from build123d import *

# Parameters (mm, degrees)
F0_W      = 43.6
F0_H      = 122.8
F1_DEPTH  = 6.1
F2_T      = -2
F3_R      = 3.5
F3_R_2    = 1.3
F4_DEPTH  = 2.5
F5_DEPTH  = 2.001
F6_W      = 1.5
F6_H      = 108.8
F6_W_2    = 5
F7_DEPTH  = 2.5
F8_W      = 5
F8_H      = 10
F9_DEPTH  = 1.5
F10_W     = 3
F10_H     = 10
F11_DEPTH = 25
F11_TAPER = -10
F0_W_2    = 5.5
F12_DEPTH = 4
F14_DEPTH = 15
F16_W     = 10
F16_H     = 3.6
F17_DEPTH = 11


with BuildPart() as f1:
    # F0 (on Top) → F1 (new body)
    with BuildSketch(Plane.XY):
        with Locations((-27.3, 0)):
            Rectangle(F0_W, F0_H)
    extrude(amount=F1_DEPTH)

    # F2
    f2_openings = [f1.faces().sort_by_distance(p)[0] for p in [
        (-27.3, 0, 6.1),
    ]]
    offset(amount=F2_T, openings=f2_openings)

    # F3 (on face) → F4 (join, through all)
    with BuildSketch(Plane.XY.offset(2)):
        with Locations((-42.45, 54.75)):
            Circle(F3_R)
        with Locations((-42.45, 54.75)):
            Circle(F3_R_2, mode=Mode.SUBTRACT)
        with Locations((-41.95, -48.25)):
            Circle(F3_R)
        with Locations((-41.95, -48.25)):
            Circle(F3_R_2, mode=Mode.SUBTRACT)
    extrude(amount=F4_DEPTH)

    # F5 (cut, through all): faces of the model
    f5_faces = [f1.faces().sort_by_distance(p)[0] for p in [
        (-42.45, 54.75, 2),
        (-41.95, -48.25, 2),
    ]]
    extrude(f5_faces, amount=-F5_DEPTH, mode=Mode.SUBTRACT)

    # F6 (on face) → F7 (join, through all)
    with BuildSketch(Plane.XY.offset(2)):
        with Locations((-46.35, -5)):
            Rectangle(F6_W, F6_H)
        with Locations((-10, -5)):
            Rectangle(F6_W_2, F6_H)
    extrude(amount=F7_DEPTH)

    # F8 (on face) → F9 (join)
    with BuildSketch(Plane.XY.offset(6.1)):
        with Locations((-8, 14.4)):
            Rectangle(F8_W, F8_H)
        with Locations((-8, -45.6)):
            Rectangle(F8_W, F8_H)
    extrude(amount=F9_DEPTH)

    # F10 (on face) → F11 (cut)
    with BuildSketch(Plane(origin=(0, 0, 6.1), x_dir=(1, 0, 0), z_dir=(0, 0, -1))):
        with Locations((-9, -14.4)):
            Rectangle(F10_W, F10_H)
        with Locations((-9, 45.6)):
            Rectangle(F10_W, F10_H)
    extrude(amount=F11_DEPTH, taper=F11_TAPER, mode=Mode.SUBTRACT)

    # F0 (on Top) → F12 (join)
    with BuildSketch(Plane.XY):
        with Locations((-2.75, 0)):
            Rectangle(F0_W_2, F0_H)
    extrude(amount=F12_DEPTH)

    # F13 (on face) → F14 (cut)
    with BuildSketch(Plane.YZ):
        with BuildLine():
            Line((49.4, 7), (49.4, 4))
            Line((49.4, 4), (49.4, 3.5))
            ThreePointArc((49.4, 3.5), (50.9, 2), (52.4, 3.5))
            Line((52.4, 3.5), (52.4, 4))
            Line((52.4, 4), (52.4, 7))
            Line((52.4, 7), (49.4, 7))
        make_face()
    extrude(amount=-F14_DEPTH, mode=Mode.SUBTRACT)

    # F15: F1 across plane


with BuildPart() as f1_1:
    add(f1.part)
    add(f1.part.mirror(Plane.YZ))

    # F16 (on face) → F17 (join, through all)
    with BuildSketch(Plane.YZ.offset(-5.5)):
        with Locations((14.4, 5.8)):
            Rectangle(F16_W, F16_H)
        with Locations((-45.6, 5.8)):
            Rectangle(F16_W, F16_H)
    extrude(amount=F17_DEPTH)


solid = f1_1.part
For this review, take the finished solid that the model builds, in its own axes (mm). A direction names the side the tool comes from. Round coordinates to 2 decimals unless told otherwise and drop trailing zeros. Loops run counter-clockwise (first coordinate to the right, second up) from the corner with the lowest first, then second, coordinate; pieces in that order, holes last. Notation, with made-up numbers: (70.5, 2) - (76.5, 2) arc R23 ccw to (76.5, 16) - close; hole circle Ø6 at (31, 76). An arc over 180 degrees is marked (long way). Put each result on its own line as item: value. Start each with the question number.
1. Consider section A-A on y = 54.75. State how many separate pieces and enclosed holes the cut face has, plus the area to 3 significant figures.
2. Consider section B-B on x = -2.5. State the section outline as (y, z) points, plus the area to 3 significant figures.
3. Insertion check: P1, Ø6, axis at x = -3, y = 57.5, coming from the +Z side; P2, Ø0.8, axis at x = -46.5, y = -13, coming from the +Z side; P3, Ø1.1, axis at x = -1.5, z = 5.5, coming from the -Y side; P4, Ø2, axis at x = -42.45, y = 54.75, coming from the -Z side. Each pin has a flat end and moves straight along its axis. Give the tip position at first contact, or say it passes through.
4. Mouldability with a two-part tool opening along X and no side actions: class faces 4 (the flat face through (-49.1, -1, 3)), 5 (the flat face through (0, 14, 7.6)), 6 (the cylindrical face through (-0.1, 50.9, 2)) as +X half, -X half, draft (parallel to the pull), parting line (faces both ways), or undercut.
5. For probe 1 along X at (y, z) = (0, 4.75); probe 2 along X at (y, z) = (-14.5, 4.25); probe 3 along Y at (x, z) = (34, 3.75), list the stretches that pass through material, from the lowest coordinate up. Write a range as [from, to].
6. Consider section D-D on y = 41. State the section outline as (x, z) points, plus the area to 3 significant figures.
7. For faces 1 (the flat face through (28, 1, 2)), 2 (the flat face through (0, 35, 4)), 3 (the flat face through (9, -46, 6.1)), list the 3-axis set-ups (+Z, -Z, +X, -X, +Y, -Y) from which the entire face can be reached by the end or side of a thin tool; tool diameter is ignored.
Result sheet:
1. separate pieces: 3
1. enclosed holes: 0
1. area: 263 mm^2
2. outline: (-61.4, 0) - (61.4, 0) - (61.4, 4) - (52.4, 4) - (52.4, 3.5) arc R1.5 cw to (49.4, 3.5) - (49.4, 4) - (19.4, 4) - (19.4, 7.6) - (9.4, 7.6) - (9.4, 4) - (-40.6, 4) - (-40.6, 7.6) - (-50.6, 7.6) - (-50.6, 4) - (-61.4, 4) - close
2. area: 558 mm^2
3. P1: z = 6.1
3. P2: z = 4.5
3. P3: y = -50.6
3. P4: through
4. face 4: -X half
4. face 5: draft
4. face 6: undercut
5. probe 1: [-49.1, -47.1], [-7.5, -5.5], [5.5, 7.5], [47.1, 49.1]
5. probe 2: [-49.1, -45.6], [-12.5, -5.5], [5.5, 12.5], [45.6, 49.1]
5. probe 3: [-61.4, -59.4], [59.4, 61.4]
6. outline: (-49.1, 0) - (49.1, 0) - (49.1, 6.1) - (47.1, 6.1) - (47.1, 4.5) - (45.6, 4.5) - (45.6, 2) - (12.5, 2) - (12.5, 4.5) - (7.5, 4.5) - (7.5, 6.1) - (5.5, 6.1) - (5.5, 4) - (-5.5, 4) - (-5.5, 6.1) - (-7.5, 6.1) - (-7.5, 4.5) - (-12.5, 4.5) - (-12.5, 2) - (-45.6, 2) - (-45.6, 4.5) - (-47.1, 4.5) - (-47.1, 6.1) - (-49.1, 6.1) - close
6. area: 284 mm^2
7. face 1: +Z
7. face 2: +Z, +Y
7. face 3: -Z
